Geometry: see drawing. Coordinates: mm, zero at the bounding-box minimum. A direction names the side the tool comes from. Give positions to 0.01 mm unless a question says otherwise; leave off trailing zeros. Order: outer loops, then holes, each group sorted by start corner. A loop starts at its lowest first (then second) coordinate and runs counter-clockwise, first axis right, second up. Notation, with made-up numbers: M -29.75,-26 L 13.25,-26 A24 ccw 13.25,-4 Z; hole C 28,-15 d10. An arc over 180 degrees is marked long. Return JSON: item names as keys, results as strings.
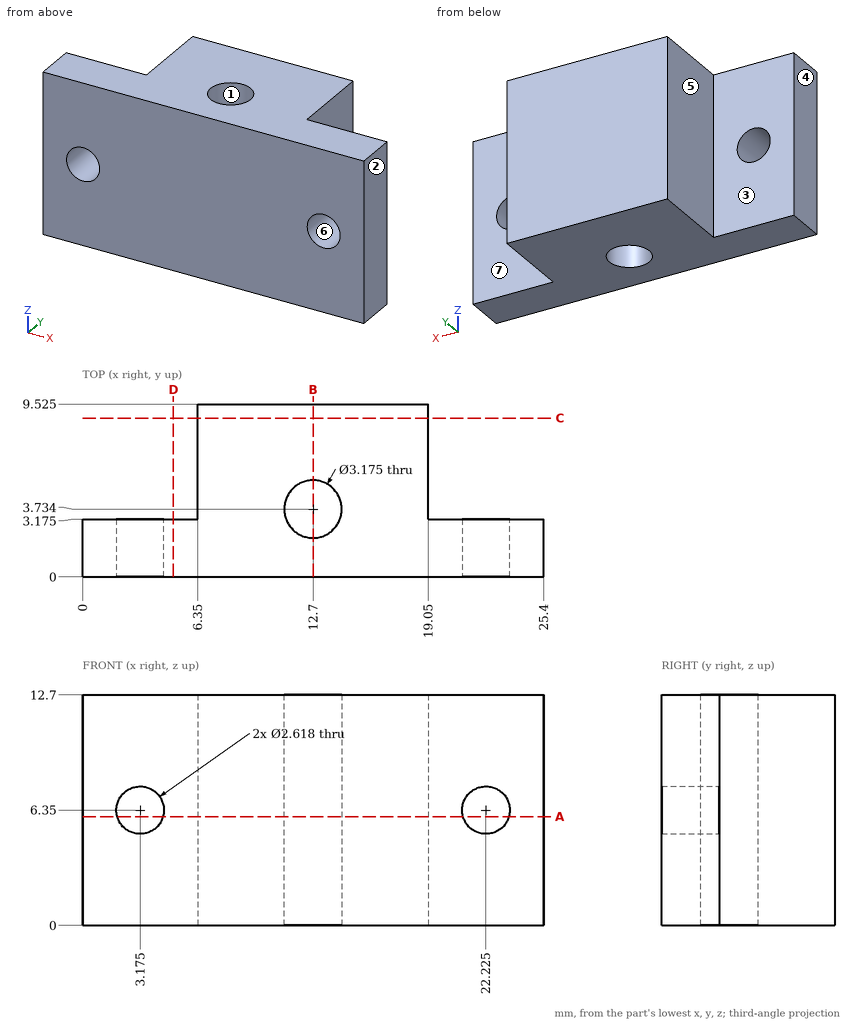
1. Section query B-B (x = 12.7). Return loops of the section in (y, z) (1 decimal).
Evaluation:
{"outline": "M 0,0 L 2.1,0 L 2.1,12.7 L 0,12.7 Z; M 5.3,0 L 9.5,0 L 9.5,12.7 L 5.3,12.7 Z"}
2. Section query A-A (z = 6). State how many separate pieces and enclosed holes the cut face has, then the cut area to 3 significant figures.
Evaluation:
{"separate pieces": "3", "enclosed holes": "1", "area": "137 mm^2"}
3. Section query C-C (y = 8.75). Return loops of the section in (x, z).
Evaluation:
{"outline": "M 6.35,0 L 19.05,0 L 19.05,12.7 L 6.35,12.7 Z"}
4. Draft query along X for the marked faces 1, 2, 3 and 4. Return one class per face: pulls with the +X half, pulls with the -X half, needs draft (parallel to the pull), parting line crosses it, or undercut.
Evaluation:
{"face 1": "undercut", "face 2": "pulls with the +X half", "face 3": "needs draft", "face 4": "pulls with the -X half"}
5. Set-up query: the marked faces 5, 6 and 7. Return all of +Z, -Z, +X, -X, +Y, -Y with unobstructed straight access to the full face (end or side cutting, diameter ignored); none if empty.
Evaluation:
{"face 5": "+Z, -Z, -X, +Y", "face 6": "+Y, -Y", "face 7": "+Z, -Z, +X, +Y"}
6. Ray query, probe 1 along Y at (x, z) = (12.7, 6.25) (1 decimal); probe 2 along X at (y, z) = (3.75, 1.5); probe 3 along Y at (x, z) = (2.25, 2) (1 decimal). Return the intervals inside material, ascending.
Evaluation:
{"probe 1": "y = 0 to 2.1, 5.3 to 9.5", "probe 2": "x = 6.35 to 11.11, 14.29 to 19.05", "probe 3": "y = 0 to 3.2"}
7. First-contact query: pin 1 (5 mm diameter, centred on x = 23, z = 8.5, fed in from +Y) (3 decimals); pin 2 (5 mm diameter, centred on y = 6, z = 3.5, fed in from +X). Flat tips, straight axial feed; report the tip coordinate or a pass-through.
Evaluation:
{"pin 1": "stops at y = 3.175", "pin 2": "stops at x = 19.05"}
8. Section query D-D (x = 5). Return loops of the section in (y, z) (1 decimal).
Evaluation:
{"outline": "M 0,0 L 3.2,0 L 3.2,12.7 L 0,12.7 Z"}
